Read the model definition and answer for the solid it produces. Units are mm, in the model's axes. Give positions to 0.01 mm unless a question says otherwise; leave off trailing zeros. Loops run counter-clockwise (first coordinate to the right, second up) from the corner with the lowest first, then second, coordinate; pieces in that order, holes last. Notation, with made-up numbers: (24, 32) - (56, 32) arc R27 cw to (56, 56) - close; hole circle Ø5 at (86.25, 60). An arc over 180 degrees is marked (long way). Write each question's results on one line, items separated by ' | '. Start each with the question number.
Q1. The part is cut by section A-A, the plane y = 12. Write down the section's boundary in (x, z), plus the area to 3 significant figures.
Q2. The part is cut by section C-C, the plane z = 0. Write down the section's boundary in (x, y).
Q3. Find the intervals of material crossed by line 1 (Y direction, x = -6.25, z = -0.5); line 2 (X direction, y = -77, z = 1), in increasing order. Write a range as from..to.
Q4. Given pin 1 (5 mm diameter, centred on y = -149, z = 4.5, fed in from +X); pin 2 (1 mm diameter, centred on x = 0.5, y = 125, fed in from +Z); pin 3 (2 mm diameter, centred on x = -5, z = 2.5, fed in from +Y), each flat-ended and moving along its own axis, determine where each tip first touches the part or whether it passes through.
Q5. The part is cut by section B-B, the plane x = 0. Write down the section's boundary in (y, z).
```python
from build123d import *

# Parameters (mm, degrees)
SKETCH_2_R      = 5
EXTRUDE_1_DEPTH = 250


with BuildPart() as part:
    # 草图2 → 凸台-拉伸1 (new, symmetric)
    with BuildSketch(Plane(origin=(0, 0, 0), x_dir=(1, 0, 0), z_dir=(0, 1, 0))):
        with Locations(Location((0, 0, 0), (0, 0, 270))):
            Circle(SKETCH_2_R)
    extrude(amount=EXTRUDE_1_DEPTH, both=True)

    # 草图3 → 旋转1 (revolve)
    with BuildSketch(Plane.XY):
        with BuildLine():
            Line((0, 257.5), (0, 242.5))
            ThreePointArc((0, 242.5), (7.5, 250), (0, 257.5))
        make_face()
    revolve_1 = revolve(axis=Axis((0, 257.5, 0), (0, -1, 0)))

    # 镜向1: 旋转1 across plane
    add(revolve_1.mirror(Plane.ZX))


solid = part.part
```
Check sheet entries:
1) outline: circle Ø10 at (0, 0) | area: 78.5 mm^2
2) outline: (-5, -244.41) arc R7.5 ccw (long way) to (5, -244.41) - (5, 244.41) arc R7.5 ccw (long way) to (-5, 244.41) - close
3) line 1: y = -254.12..-245.88, 245.88..254.12 | line 2: x = -4.9..4.9
4) pin 1: stops at x = 4.58 | pin 2: stops at z = 5 | pin 3: stops at y = 255.93
5) outline: (-244.41, -5) - (244.41, -5) arc R7.5 ccw (long way) to (244.41, 5) - (-244.41, 5) arc R7.5 ccw (long way) to start
